Can you work these out from the model? Positions are in its coordinate system, mm. A direction names the side the tool comes from. Coordinates: 2 decimals unless noted, no trailing zeros. Order: outer loops, then holes, each group sorted by start corner. A loop starts at its lowest first (then second) coordinate and runs counter-clockwise, first axis right, second up. Notation, with made-up numbers: (16, 88) -> (65, 88) arc R16 cw to (65, 99) -> close; hole circle Ø11 at (59, -2.75). An arc over 180 degrees is marked (long way). Write item = value, one per line. Start each with the question number.
from build123d import *

# Parameters (mm, degrees)
SKETCH2_W               = 27
SKETCH2_H               = 49
SKETCH2_R               = 2.05
BOSS_EXTRUDE1_DEPTH     = 3
BOSS_EXTRUDE2_DEPTH     = 49
SKETCH5_R               = 4.5
CUT_EXTRUDE1_DEPTH      = 4
FILLET1_R               = 1
SKETCH6_W               = 13.2
SKETCH6_H               = 5
CUT_EXTRUDE2_DEPTH      = 4
SKETCH7_W               = 10.2
SKETCH7_H               = 5
CUT_EXTRUDE3_DEPTH      = 28
CUT_EXTRUDE3_DEPTH_BACK = 4


with BuildPart() as part:
    # Sketch2 → Boss-Extrude1 (new body)
    with BuildSketch(Plane.XY):
        with Locations((13.5, 24.5)):
            Rectangle(SKETCH2_W, SKETCH2_H)
        with Locations((6, 39)):
            Circle(SKETCH2_R, mode=Mode.SUBTRACT)
        with Locations((21, 39)):
            Circle(SKETCH2_R, mode=Mode.SUBTRACT)
        with Locations((6, 10)):
            Circle(SKETCH2_R, mode=Mode.SUBTRACT)
        with Locations((21, 10)):
            Circle(SKETCH2_R, mode=Mode.SUBTRACT)
    extrude(amount=BOSS_EXTRUDE1_DEPTH)

    # Sketch4 → Boss-Extrude2 (add)
    with BuildSketch(Plane(origin=(0, 49, 0), x_dir=(1, 0, 0), z_dir=(0, 1, 0))):
        with BuildLine():
            Line((30, -3), (30, -33))
            Line((30, -33), (27, -33))
            Line((27, -33), (27, 0))
            ThreePointArc((27, 0), (29.121320344, -0.878679656), (30, -3))
        make_face()
    extrude(amount=-BOSS_EXTRUDE2_DEPTH)

    # Sketch5 → Cut-Extrude1 (cut, through all)
    with BuildSketch(Plane.ZY.offset(-27)):
        with Locations((18, 39)):
            Circle(SKETCH5_R)
        with Locations((18, 10)):
            Circle(SKETCH5_R)
    extrude(amount=-CUT_EXTRUDE1_DEPTH, mode=Mode.SUBTRACT)

    # Fillet1
    fillet1_edges = [part.edges().sort_by_distance(p)[0] for p in [
        (27, 24.5, 3),
    ]]
    fillet(fillet1_edges, radius=FILLET1_R)

    # Sketch6 → Cut-Extrude2 (cut, through all)
    with BuildSketch(Plane.XY.offset(3)):
        with Locations((3.6, 24.5)):
            Rectangle(SKETCH6_W, SKETCH6_H)
    extrude(amount=-CUT_EXTRUDE2_DEPTH, mode=Mode.SUBTRACT)

    # Sketch7 → Cut-Extrude3 (cut, two sides)
    with BuildSketch(Plane.ZY.offset(-27)) as cut_extrude3_sk:
        with Locations((27.9, 24.5)):
            Rectangle(SKETCH7_W, SKETCH7_H)
    extrude(amount=CUT_EXTRUDE3_DEPTH, mode=Mode.SUBTRACT)
    extrude(cut_extrude3_sk.sketch, amount=-CUT_EXTRUDE3_DEPTH_BACK, mode=Mode.SUBTRACT)


solid = part.part
(1) Thinking about a two-plate mould opening in Y: for faces 5 (the face through (5.733, 41.033, 1.479)), 6 (the face through (27.3, 49, 9.1)), 7 (the face through (13, 25, 3)), which applies, +Y half, -Y half, draft (parallel to the pull), parting line (faces both ways), or undercut?
(2) Imagine slicing it at C-C (x = 6). Write out the boundary of the cut face in (y, z), plus the area to 3 significant figures.
(3) Imagine slicing it at A-A (z = 18). Write out the boundary of the cut face in (x, y), plus the area to 3 significant figures.
(4) Imagine slicing it at B-B (z = 27). Write out the boundary of the cut face in (x, y), plus the area to 3 significant figures.
(5) If I drill on L1, parallel to Y at x = 28.15, z = 18; L2, parallel to Y at x = 21, z = 0.7; L3, parallel to Y at x = 6, z = 2.2, over which ranges is the centre line in solid material (lowest first)? Write a range as from..to.
(6) For faces 1 (the face through (28, 22, 28)), 2 (the face through (5, 27, 2)), 3 (the face through (27, 25, 19)), 4 (the face through (30, 25, 18)), which set-ups out of +Z, -Z, +X, -X, +Y, -Y let a thin tool reach every point of the face, with its end or its side?
(7) For P1, Ø10.5, axis at y = 10, z = 18, coming from the +X side; P2, Ø5, axis at x = 24, y = 39.5, coming from the +Z side; P3, Ø5.5, axis at x = 6, y = 39, coming from the +Z side; P4, Ø0.9, axis at y = 24, z = 1.5, coming from the -X side, each with a flat end and sliding along its axis, tell me the tip position at first contact or that it passes through.
(8) Imagine slicing it at D-D (y = 39). Write out the boundary of the cut face in (x, z).
Result set:
q1.face_5 = undercut
q1.face_6 = +Y half
q1.face_7 = draft
q2.outline = (0, 0) -> (7.95, 0) -> (7.95, 3) -> (0, 3) -> close; (12.05, 0) -> (22, 0) -> (22, 3) -> (12.05, 3) -> close; (27, 0) -> (36.95, 0) -> (36.95, 3) -> (27, 3) -> close; (41.05, 0) -> (49, 0) -> (49, 3) -> (41.05, 3) -> close
q2.area = 107 mm2
q3.outline = (27, 0) -> (30, 0) -> (30, 5.5) -> (27, 5.5) -> close; (27, 14.5) -> (30, 14.5) -> (30, 34.5) -> (27, 34.5) -> close; (27, 43.5) -> (30, 43.5) -> (30, 49) -> (27, 49) -> close
q3.area = 93.0 mm2
q4.outline = (27, 0) -> (30, 0) -> (30, 22) -> (27, 22) -> close; (27, 27) -> (30, 27) -> (30, 49) -> (27, 49) -> close
q4.area = 132 mm2
q5.L1 = 0..5.5, 14.5..34.5, 43.5..49
q5.L2 = 0..7.95, 12.05..36.95, 41.05..49
q5.L3 = 0..7.95, 12.05..22, 27..36.95, 41.05..49
q6.face_1 = +Z, +X, -X
q6.face_2 = +Z, -Z, -X
q6.face_3 = +Z, -X, +Y, -Y
q6.face_4 = +Z, -Z, +X, +Y, -Y
q7.P1 = 30
q7.P2 = 3.13
q7.P3 = 3
q7.P4 = 10.2
q8.outline = (0, 0) -> (3.95, 0) -> (3.95, 3) -> (0, 3) -> close; (8.05, 0) -> (18.95, 0) -> (18.95, 3) -> (8.05, 3) -> close; (23.05, 0) -> (27, 0) arc R3 ccw to (30, 3) -> (30, 13.5) -> (27, 13.5) -> (27, 4) arc R1 cw to (26, 3) -> (23.05, 3) -> close; (27, 22.5) -> (30, 22.5) -> (30, 33) -> (27, 33) -> close
